Read the model definition and answer for the solid it produces. Units are mm, in the model's axes. A direction names the side the tool comes from. Coordinates: 2 decimals unless noted, no trailing zeros. Loops run counter-clockwise (first coordinate to the right, second up) from the corner with the lowest first, then second, coordinate; pieces in that order, holes last.
from build123d import *

# Parameters (mm, degrees)
SZKIC1_R                    = 4.25
SZKIC1_R_2                  = 0.635
SZKIC1_R_3                  = 3
DODANIE_WYCI_GNI_CIE1_DEPTH = 5
SZKIC1_2_R                  = 3
DODANIE_WYCI_GNI_CIE2_DEPTH = 15


with BuildPart() as part:
    # Szkic1 → Dodanie-wyci_gni_cie1 (new body)
    with BuildSketch(Plane.XY):
        with BuildLine():
            Line((-50.67287635, 5.055665151), (-9.235111676, 10.570763761))
            ThreePointArc((-9.235111676, 10.570763761), (0, 11.182632843), (9.235111676, 10.570763761))
            Line((9.235111676, 10.570763761), (50.67287635, 5.055665151))
            ThreePointArc((50.67287635, 5.055665151), (55.100246338, 0), (50.67287635, -5.055665151))
            Line((50.67287635, -5.055665151), (9.235111676, -10.570763761))
            ThreePointArc((9.235111676, -10.570763761), (0, -11.182632843), (-9.235111676, -10.570763761))
            Line((-9.235111676, -10.570763761), (-50.67287635, -5.055665151))
            ThreePointArc((-50.67287635, -5.055665151), (-55.100246338, 0), (-50.67287635, 5.055665151))
        make_face()
        Circle(SZKIC1_R, mode=Mode.SUBTRACT)
        with Locations((-5.656854249, 5.656854249)):
            Circle(SZKIC1_R_2, mode=Mode.SUBTRACT)
        with Locations((-8, 0)):
            Circle(SZKIC1_R_2, mode=Mode.SUBTRACT)
        with Locations((0, 8)):
            Circle(SZKIC1_R_2, mode=Mode.SUBTRACT)
        with Locations((5.656854249, 5.656854249)):
            Circle(SZKIC1_R_2, mode=Mode.SUBTRACT)
        with Locations((-50, 0)):
            Circle(SZKIC1_R_3, mode=Mode.SUBTRACT)
        with Locations((50, 0)):
            Circle(SZKIC1_R_3, mode=Mode.SUBTRACT)
        with Locations((8, 0)):
            Circle(SZKIC1_R_2, mode=Mode.SUBTRACT)
        with Locations((5.656854249, -5.656854249)):
            Circle(SZKIC1_R_2, mode=Mode.SUBTRACT)
        with Locations((0, -8)):
            Circle(SZKIC1_R_2, mode=Mode.SUBTRACT)
        with Locations((-5.656854249, -5.656854249)):
            Circle(SZKIC1_R_2, mode=Mode.SUBTRACT)
    extrude(amount=DODANIE_WYCI_GNI_CIE1_DEPTH)

    # Szkic1_2 → Dodanie-wyci_gni_cie2 (add)
    with BuildSketch(Plane.XY):
        with Locations((-50, 0)):
            Circle(SZKIC1_2_R)
        with Locations((50, 0)):
            Circle(SZKIC1_2_R)
    extrude(amount=DODANIE_WYCI_GNI_CIE2_DEPTH)


solid = part.part
Q1. A cutting plane is placed at B-B (z = 11). Give the vertices of the cut face in (x, y), then the cut area to 3 significant figures.
Findings below:
outline: circle Ø6 at (-50, 0); circle Ø6 at (50, 0)
area: 56.5 mm2
Q2. Which of the six approach directions +Z, -Z, +X, -X, +Y, -Y give full straight-line access (tool end or side, diameter ignored) to faces 4 (the face through (-55.1, -0.1, 2.5)), 5 (the face through (-53, 0, 10))?
Findings below:
face 4: +Z, -Z, -X
face 5: +Z
Q3. Straight lines are drawn through the part: probe 1 along Y at (x, z) = (0, 2.7) (3 decimals); probe 2 along Z at (x, y) = (47, 5.5); probe 3 along Y at (x, z) = (8, 2.8) (3 decimals). For each, find the intervals that lie inside material, in ascending order.
Findings below:
probe 1: y = -11.183 to -8.635, -7.365 to -4.25, 4.25 to 7.365, 8.635 to 11.183
probe 2: z = 0 to 5
probe 3: y = -10.724 to -0.635, 0.635 to 10.724
Q4. A cutting plane is placed at C-C (x = 39.5). Give the vertices of the cut face in (y, z).
Findings below:
outline: (-6.54, 0) - (6.54, 0) - (6.54, 5) - (-6.54, 5) - close
Q5. A cutting plane is placed at A-A (z = 3). Count the separate pieces of the cut face and the enclosed holes in it, then the cut area to 3 significant figures.
Findings below:
separate pieces: 1
enclosed holes: 9
area: 1,700 mm2
Q6. Determine the mould class of faces 1 (the face through (-30.244, 7.775, 2.465)), 2 (the face through (1, -5, 0)), 3 (the face through (47, 0, 10)) for opening direction X: +X half, -X half, draft (parallel to the pull), parting line (faces both ways), or undercut.
Findings below:
face 1: -X half
face 2: draft
face 3: undercut
Q7. Flat-ended cylindrical pins translate along their axes: pin 1 Ø5 at (x, y) = (26.5, -1.5) entering from +Z; pin 2 Ø1.5 at (x, z) = (14.5, 3) entering from +Y; pin 3 Ø4 at (y, z) = (-1, 10.5) entering from -X; pin 4 Ø1.7 at (x, y) = (-5.66, -5.66) entering from -Z. Find the tip coordinate at first contact, or state that the pin passes through.
Findings below:
pin 1: stops at z = 5
pin 2: stops at y = 9.97
pin 3: stops at x = -53
pin 4: stops at z = 0
